Verification items for the finished model (mm, model axes). A direction names the side the tool comes from. Coordinates: 2 decimals unless noted, no trailing zeros. Order: outer loops, then holes, each group sorted by start corner. A loop starts at its lowest first (then second) coordinate and runs counter-clockwise, first axis right, second up. Notation, with made-up numbers: M 5,38 L 40,38 A22 ccw 40,66 Z; hole C 72.5,47.5 d9. An arc over 180 degrees is marked long. Return JSON: item names as keys, results as strings. Group by question number.
Q1. Section check A-A, the plane y = 1.45. Enter the section's corners in (x, z).
Q2. Go/stop test with flat-tipped pins: pin 1 Ø0.6 at (y, z) = (1, -36.5) entering from -X; pin 2 Ø0.6 at (x, y) = (14, 1.5) entering from -Z. Record where each tip stops, or that it passes through.
Q3. Section check C-C, the plane x = 4.5. Enter the section's corners in (y, z).
Q4. Thickness scan on probe 1 along Z at (x, y) = (10.5, 1); probe 2 along Z at (x, y) = (13, 1.35); probe 3 along X at (y, z) = (0.7, -17). Record the ranges inside material, lowest first.
Q5. Mould release check, pull along X, two halves, no side actions. Record for faces 5 (the face through (9, 2, -13)), 6 (the face through (12.6, 1, -18)), 7 (the face through (12.6, 1, 1)): pulls with the +X half, pulls with the -X half, needs draft (parallel to the pull), parting line crosses it, or undercut.
Q6. Access from +Z, -Z, +X, -X, +Y, -Y to the whole of each face (thin tool, end or side, straight path). Record for faces 1 (the face through (5, 1, -36)), 2 (the face through (2, 1, 0)), 3 (the face through (15, 1, 0)), 4 (the face through (9, 1, -16.8)).
Q7. Section check B-B, the plane x = 7.25. Enter the section's corners in (y, z).
from build123d import *

# Parameters (mm, degrees)
SKETCH_1_W      = 17.6
SKETCH_1_H      = 34.8
SKETCH_1_W_2    = 7.6
SKETCH_1_H_2    = 2.2
SKETCH_1_H_3    = 2
EXTRUDE_1_DEPTH = 2


with BuildPart() as part:
    # 草图1 → 凸台-拉伸1 (new body)
    with BuildSketch(Plane(origin=(0, 0, 0), x_dir=(1, 0, 0), z_dir=(0, 1, 0))):
        with Locations((8.8, 17.4)):
            Rectangle(SKETCH_1_W, SKETCH_1_H)
        with Locations((8.8, 17.9)):
            Rectangle(SKETCH_1_W_2, SKETCH_1_H_2, mode=Mode.SUBTRACT)
        with Locations((8.8, -1)):
            Rectangle(SKETCH_1_W_2, SKETCH_1_H_3)
        with Locations((8.8, 35.8)):
            Rectangle(SKETCH_1_W_2, SKETCH_1_H_3)
    extrude(amount=EXTRUDE_1_DEPTH)


solid = part.part
Numbers:
{
 "1": {"outline": "M 0,-34.8 L 5,-34.8 L 5,-36.8 L 12.6,-36.8 L 12.6,-34.8 L 17.6,-34.8 L 17.6,0 L 12.6,0 L 12.6,2 L 5,2 L 5,0 L 0,0 Z; hole M 5,-19 L 12.6,-19 L 12.6,-16.8 L 5,-16.8 Z"},
 "2": {"pin 1": "stops at x = 5", "pin 2": "stops at z = -34.8"},
 "3": {"outline": "M 0,-34.8 L 2,-34.8 L 2,0 L 0,0 Z"},
 "4": {"probe 1": "z = -36.8 to -19, -16.8 to 2", "probe 2": "z = -34.8 to 0", "probe 3": "x = 0 to 5, 12.6 to 17.6"},
 "5": {"face 5": "needs draft", "face 6": "undercut", "face 7": "pulls with the +X half"},
 "6": {"face 1": "-Z, -X, +Y, -Y", "face 2": "+Z, -X, +Y, -Y", "face 3": "+Z, +X, +Y, -Y", "face 4": "+Y, -Y"},
 "7": {"outline": "M 0,-36.8 L 2,-36.8 L 2,-19 L 0,-19 Z; M 0,-16.8 L 2,-16.8 L 2,2 L 0,2 Z"}
}
